Autodesk Inventor part; units mm, degrees
ref_plane "YZ Plane" through (0, 0, 0) normal (1, 0, 0) x (0, 1, 0)
ref_plane "XZ Plane" through (0, 0, 0) normal (0, 1, 0) x (-1, 0, 0)
ref_plane "XY Plane" through (0, 0, 0) normal (0, 0, 1) x (1, 0, 0)
sketch "Schizzo1" plane through (0, 0, 0) normal (0, 1, 0) x (-1, 0, 0)
  line L0 (0, 0) -> (320, 0)
  line L1 (320, 0) -> (320, -415)
  line L2 (320, -415) -> (0, -415)
  line L3 (0, -415) -> (0, 0)
  dimension "d0" = 320
  dimension "d1" = 415
extrude "Estrusione1" add sketch "Schizzo1" along normal blind 4
chamfer "Smusso1" distance 10 angle 45 4 edges at (0, 2, 0) (0, 2, -415) (-320, 2, -415) (-320, 2, 0)
sketch "Schizzo2" plane through (0, 4, 0) normal (0, 1, 0) x (1, 0, 0)
  line L0 (-306, 14) -> (-14, 14) construction
  line L1 (-14, 14) -> (-14, 401)
  line L2 (-14, 401) -> (-306, 401) construction
  line L3 (-306, 401) -> (-306, 14) construction
  line L4 (-320, 405) -> (-320, 10)
  line L5 (-10, 415) -> (-310, 415)
  point P0 (0, 0)
  point P1 (-306, 207.5)
  point P2 (-320, 207.5)
  point P3 (-160, 401)
  point P4 (-160, 415)
  point P5 (-306, 62.375)
  point P6 (-306, 110.75)
  point P7 (-306, 159.125)
  point P8 (-306, 207.5)
  point P9 (-306, 255.875)
  point P10 (-306, 304.25)
  point P11 (-306, 352.625)
  point P12 (-14, 62.375)
  point P13 (-14, 110.75)
  point P14 (-14, 159.125)
  point P15 (-14, 207.5)
  point P16 (-14, 255.875)
  point P17 (-14, 304.25)
  point P18 (-14, 352.625)
  point P19 (-257.3333, 401)
  point P20 (-208.6667, 401)
  point P21 (-160, 401)
  point P22 (-111.3333, 401)
  point P23 (-62.6667, 401)
  point P24 (-257.3333, 14)
  point P25 (-208.6667, 14)
  point P26 (-160, 14)
  point P27 (-111.3333, 14)
  point P28 (-62.6667, 14)
  dimension "d7" = 387
  dimension "d8" = 292
  dimension "d11" = 48.375
  dimension "d18" = 48.375
  dimension "d25" = 48.6667
  dimension "d32" = 48.6667
hole "Foro1" at (-306, 4, -14) at (-14, 4, -14) at (-14, 4, -401) at (-306, 4, -401) at (-306, 4, -62.375) at (-306, 4, -110.75) at (-306, 4, -159.125) at (-306, 4, -207.5) at (-306, 4, -255.875) at (-306, 4, -304.25) at (-306, 4, -352.625) at (-14, 4, -62.375) at (-14, 4, -110.75) at (-14, 4, -159.125) at (-14, 4, -207.5) at (-14, 4, -255.875) at (-14, 4, -304.25) at (-14, 4, -352.625) at (-257.3333, 4, -401) at (-208.6667, 4, -401) at (-160, 4, -401) at (-111.3333, 4, -401) at (-62.6667, 4, -401) at (-257.3333, 4, -14) at (-208.6667, 4, -14) at (-160, 4, -14) at (-111.3333, 4, -14) at (-62.6667, 4, -14) direction (0, -1, 0) diameter 5 end through all
sketch "Schizzo3" plane through (0, 4, 0) normal (0, 1, 0) x (1, 0, 0)
  line L0 (0, 10) -> (0, 405)
  line L1 (-310, 0) -> (-10, 0)
  line L2 (-10, 415) -> (-310, 415)
  point P0 (0, 0)
  point P1 (-50, 65)
  point P2 (-50, 350)
  dimension "d44" = 50
  dimension "d45" = 65
  dimension "d46" = 65
hole "Foro2" at (-50, 4, -65) at (-50, 4, -350) direction (0, -1, 0) diameter 7 end through all
sketch "Schizzo4" plane through (0, 4, 0) normal (0, 1, 0) x (1, 0, 0)
  line L0 (-10, 415) -> (-310, 415)
  line L1 (-320, 405) -> (-320, 10)
  circle A0 centre (-215, 310) radius 12.5
  arc A1 (-187.5, 318.6603) -> (-177.5, 318.6603) centre (-182.5, 310) ccw
  line L2 (-187.5, 318.6603) -> (-177.5, 318.6603)
  arc A2 (-155, 318.6603) -> (-145, 318.6603) centre (-150, 310) ccw
  line L3 (-155, 318.6603) -> (-145, 318.6603)
  arc A3 (-122.5, 318.6603) -> (-112.5, 318.6603) centre (-117.5, 310) ccw
  line L4 (-122.5, 318.6603) -> (-112.5, 318.6603)
  arc A4 (-90, 318.6603) -> (-80, 318.6603) centre (-85, 310) ccw
  line L5 (-90, 318.6603) -> (-80, 318.6603)
  point P0 (0, 0)
  point P1 (-52.5, 310)
  dimension "d54" = 105
  dimension "d55" = 105
  dimension "d58" = 32.5
  dimension "d63" = 25
  dimension "d64" = 20
  dimension "d65" = 10
  dimension "d70" = 20
  dimension "d71" = 10
  dimension "d76" = 20
  dimension "d77" = 10
  dimension "d88" = 20
  dimension "d89" = 10
extrude "Estrusione3" cut sketch "Schizzo4" against normal blind 4
sketch "Schizzo5" plane through (0, 4, 0) normal (0, 1, 0) x (1, 0, 0)
  circle A0 centre (-215, 310) radius 12.5
  line L0 (-10, 415) -> (-310, 415)
  arc A1 (-217.5, 357.0711) -> (-212.5, 357.0711) centre (-215, 350) ccw
  line L1 (-217.5, 357.0711) -> (-212.5, 357.0711)
  arc A2 (-185, 357.0711) -> (-180, 357.0711) centre (-182.5, 350) ccw
  line L2 (-185, 357.0711) -> (-180, 357.0711)
  arc A3 (-87.5, 357.0711) -> (-82.5, 357.0711) centre (-85, 350) ccw
  line L3 (-87.5, 357.0711) -> (-82.5, 357.0711)
  arc A4 (-120, 357.0711) -> (-115, 357.0711) centre (-117.5, 350) ccw
  line L4 (-120, 357.0711) -> (-115, 357.0711)
  arc A5 (-152.5, 357.0711) -> (-147.5, 357.0711) centre (-150, 350) ccw
  line L5 (-152.5, 357.0711) -> (-147.5, 357.0711)
  point P0 (0, 0)
  dimension "d94" = 65
  dimension "d97" = 32.5
  dimension "d102" = 15
  dimension "d103" = 5
  dimension "d108" = 15
  dimension "d109" = 5
  dimension "d114" = 15
  dimension "d115" = 5
  dimension "d120" = 15
  dimension "d121" = 5
  dimension "d126" = 15
  dimension "d127" = 5
extrude "Estrusione4" cut sketch "Schizzo5" against normal blind 4 contours L1 A1 | L2 A2 | L3 A3 | L4 A4 | L5 A5
properties part number "Husky_cover_plate"
Work out the finished part from the listing and answer in its coordinate system (mm). Coordinates: 2 decimals unless noted, no trailing zeros. Use one line per item in the form item = value. Start each with the question number.
1. Straight lines are drawn through the part: probe 1 along Z at (x, y) = (-50, 2.15); probe 2 along Z at (x, y) = (-215, 2.7); probe 3 along Z at (x, y) = (-206, 0.5). For each, find the intervals that lie inside material, in ascending order. Write a range as from..to.
2. The part is cut by section A-A (y = 3.35). Give the number of separate pieces and of enclosed holes in the cut face, plus the area to 3 significant figures.
3. The mould has two halves that part along Z. Classify faces 1 (the face through (-117.866, 2.028, -300.007)), 2 (the face through (-5, 2, -410)), 3 (the face through (-182.794, 2.028, -342.506)), 4 (the face through (-5, 2, -5)): released by +Z, released by -Z, zero draft, split by the parting line, or undercut.
Evaluation:
q1.probe_1 = -415..-353.5, -346.5..-68.5, -61.5..0
q1.probe_2 = -415..-357.07, -342.5..-322.5, -297.5..0
q1.probe_3 = -415..-318.67, -301.33..0
q2.separate_pieces = 1
q2.enclosed_holes = 40
q2.area = 129,000 mm^2
q3.face_1 = undercut
q3.face_2 = released by -Z
q3.face_3 = undercut
q3.face_4 = released by +Z
